Check sheet for the modelled part. Datum: model origin and axes. Units: mm. Face numbers are marked on the shaded views. A direction names the side the tool comes from. Give positions to 0.01 mm unless a question says otherwise; leave off trailing zeros. Order: outer loops, then holes, each group sorted by start corner. A loop starts at its lowest first (then second) coordinate and runs counter-clockwise, first axis right, second up. Notation, with made-up numbers: (36.5, -10) -> (40.5, -10) arc R19 cw to (40.5, -2) -> close; hole circle Ø3 at (6, -4.5). An arc over 180 degrees is marked (long way). Answer in a Markdown table with one row per item. Add a question column.
(1) Cross-section at D-D (x = 54). Record the cut outline in (y, z), then the cut area to 3 significant figures.
(2) Cross-section at B-B (x = 40). State how many separate pieces and enclosed holes the cut face has, then the cut area to 3 significant figures.
(3) Cross-section at C-C (y = 8). Record the cut outline in (x, z).
(4) Set-up check for the marked faces 1, 2, 3 and 4: record each of +Z, -Z, +X, -X, +Y, -Y from which the full face is reachable in a straight line by a thin tool's end or side.
(5) Thickness scan on L1, parallel to Z at x = 54, y = 13.25; L2, parallel to Z at x = 74, y = 1; L3, parallel to X at y = 5, z = 5. Record the ranges inside material, lowest first. Write a range as [from, to].
(6) Cross-section at A-A (z = 5). Record the cut outline in (x, y), then the cut area to 3 significant figures.
(7) Go/stop test with flat-tipped pins: pin 1 (5.5 mm diameter, centred on x = 30, z = -21.5, fed in from +Y); pin 2 (2 mm diameter, centred on x = 28, y = -36, fed in from -Z); pin 3 (3 mm diameter, centred on x = 74.5, z = -77, fed in from -Y); pin 4 (1.5 mm diameter, centred on x = 23.5, z = -4.5, fed in from -Y). Record where each tip stops, or that it passes through.
(8) Release check for a two-part mould opening along X. For the marked faces 5, 6 and 7 record: released by +X, released by -X, zero draft, split by the parting line, or undercut.
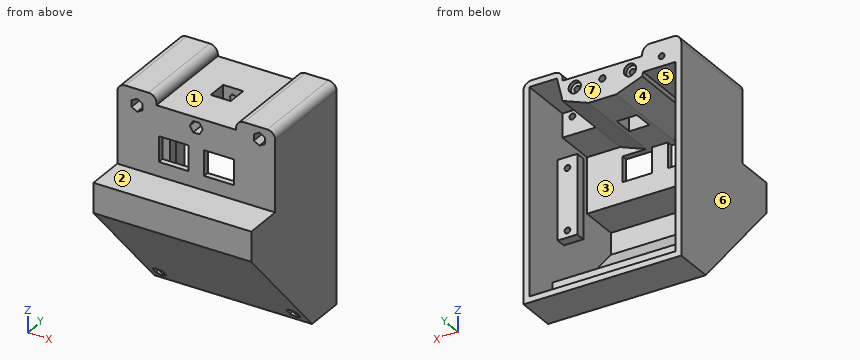
```python
from build123d import *

# Parameters (mm, degrees)
BOSS_EXTRUDE1_DEPTH = 80
SHELL1_T            = -3
SKETCH3_W           = 46
SKETCH3_H           = 47
BOSS_EXTRUDE2_DEPTH = 17
SKETCH4_W           = 10.2
SKETCH4_H           = 10.2
CUT_EXTRUDE1_DEPTH  = 20
SKETCH6_W           = 15
SKETCH6_H           = 12.8
CUT_EXTRUDE2_DEPTH  = 3
SKETCH7_W           = 40.4
SKETCH7_H           = 50
CUT_EXTRUDE3_DEPTH  = 5
FILLET1_R           = 4
CUT_EXTRUDE7_DEPTH  = 47
SKETCH13_R          = 1.5
CUT_EXTRUDE8_DEPTH  = 25
SKETCH14_R          = 3.1
CUT_EXTRUDE9_DEPTH  = 2
SKETCH17_W          = 45
SKETCH17_H          = 5
BOSS_EXTRUDE5_DEPTH = 74
CUT_EXTRUDE10_REACH = 48.51
SKETCH18_W          = 54
SKETCH18_H          = 45
CUT_EXTRUDE11_REACH = 48.51
SKETCH19_R          = 1.45
BOSS_EXTRUDE6_DEPTH = 47
SKETCH22_R          = 1.45
CUT_EXTRUDE12_DEPTH = 70.509632224
BOSS_EXTRUDE7_DEPTH = 74
SKETCH27_R          = 1.65
CUT_EXTRUDE14_DEPTH = 10
CUT_EXTRUDE15_START = -3
CUT_EXTRUDE15_DEPTH = 32
CUT_EXTRUDE16_DEPTH = 30
BOSS_EXTRUDE8_DEPTH = 20
SKETCH31_R          = 1.5
CUT_EXTRUDE17_DEPTH = 43.509632224
CUT_EXTRUDE18_DEPTH = 15
CUT_EXTRUDE19_REACH = 48.51
SKETCH33_W          = 10
SKETCH33_H          = 5
SKETCH34_R          = 1.6
CUT_EXTRUDE20_DEPTH = 70.509632224
CUT_EXTRUDE22_DEPTH = 14


with BuildPart() as part:
    # Sketch2 → Boss-Extrude1 (new body)
    with BuildSketch(Plane(origin=(0, 0, 0), x_dir=(0, 0, -1), z_dir=(1, 0, 0))):
        Polygon((-27.320490368, 20.998248687), (-27.320490368, -29.001751313), (12.679509632, -29.001751313), (12.679509632, -48.511383538), (27.679509632, -48.511383538), (82.679509632, 0.998248687), (82.679509632, 20.998248687), align=None)
    extrude(amount=BOSS_EXTRUDE1_DEPTH)

    # Shell1
    shell1_openings = [part.faces().sort_by_distance(p)[0] for p in [
        (40, 20.998248687, -27.679509632),
    ]]
    offset(amount=SHELL1_T, openings=shell1_openings, kind=Kind.INTERSECTION)

    # Sketch3 → Boss-Extrude2 (add)
    with BuildSketch(Plane(origin=(0, 0, 24.320490368), x_dir=(-1, 0, 0), z_dir=(0, 0, -1))):
        with Locations((-40, -2.501751313)):
            Rectangle(SKETCH3_W, SKETCH3_H)
    extrude(amount=BOSS_EXTRUDE2_DEPTH)

    # Sketch4 → Cut-Extrude1 (cut)
    with BuildSketch(Plane.XY.offset(27.320490368)):
        with Locations((40, -4.001751313)):
            Rectangle(SKETCH4_W, SKETCH4_H)
    extrude(amount=-CUT_EXTRUDE1_DEPTH, mode=Mode.SUBTRACT)

    # Sketch6 → Cut-Extrude2 (cut)
    with BuildSketch(Plane.XZ.offset(29.001751313)):
        with Locations((51.5, 0.920490368)):
            Rectangle(SKETCH6_W, SKETCH6_H)
        with Locations((28.5, 0.920490368)):
            Rectangle(SKETCH6_W, SKETCH6_H)
    extrude(amount=-CUT_EXTRUDE2_DEPTH, mode=Mode.SUBTRACT)

    # Sketch7 → Cut-Extrude3 (cut)
    with BuildSketch(Plane.XY.offset(27.320490368)):
        with Locations((40, -4.001751313)):
            Rectangle(SKETCH7_W, SKETCH7_H)
    extrude(amount=-CUT_EXTRUDE3_DEPTH, mode=Mode.SUBTRACT)

    # Fillet1
    fillet1_edges = [part.edges().sort_by_distance(p)[0] for p in [
        (19.8, -4.001751313, 27.320490368),
        (60.2, -4.001751313, 27.320490368),
        (80, -4.001751313, 27.320490368),
        (0, -4.001751313, 27.320490368),
    ]]
    fillet(fillet1_edges, radius=FILLET1_R)

    # Sketch12 → Cut-Extrude7 (cut)
    with BuildSketch(Plane(origin=(0, 20.998248687, 0), x_dir=(1, 0, 0), z_dir=(0, 1, 0))):
        Polygon((33, -7.320490368), (19.8, -12.320490368), (17, -24.320490368), (17, -7.320490368), align=None)
        Polygon((47, -7.320490368), (63, -7.320490368), (63, -24.320490368), (60.2, -12.320490368), align=None)
    extrude(amount=-CUT_EXTRUDE7_DEPTH, mode=Mode.SUBTRACT)

    # Sketch13 → Cut-Extrude8 (cut)
    with BuildSketch(Plane(origin=(0, 20.998248687, 0), x_dir=(1, 0, 0), z_dir=(0, 1, 0))):
        with Locations((26, -17.320490368)):
            Circle(SKETCH13_R)
        with Locations((54, -17.320490368)):
            Circle(SKETCH13_R)
    extrude(amount=-CUT_EXTRUDE8_DEPTH, mode=Mode.SUBTRACT)

    # Sketch14 → Cut-Extrude9 (cut)
    with BuildSketch(Plane(origin=(0, 20.998248687, 0), x_dir=(1, 0, 0), z_dir=(0, 1, 0))):
        with Locations((26, -17.320490368)):
            Circle(SKETCH14_R)
        with Locations((54, -17.320490368)):
            Circle(SKETCH14_R)
    extrude(amount=-CUT_EXTRUDE9_DEPTH, mode=Mode.SUBTRACT)

    # Sketch17 → Boss-Extrude5 (add)
    with BuildSketch(Plane.ZY.offset(-77)):
        with Locations((-23.179509632, -4.501751313)):
            Rectangle(SKETCH17_W, SKETCH17_H)
    extrude(amount=BOSS_EXTRUDE5_DEPTH)

    # Sketch18 → Cut-Extrude10 (cut, up to next)
    with BuildSketch(Plane(origin=(0, -2.001751313, 0), x_dir=(1, 0, 0), z_dir=(0, 1, 0)), mode=Mode.PRIVATE) as cut_extrude10_sk1:
        with Locations((40, 23.179509632)):
            Rectangle(SKETCH18_W, SKETCH18_H)
    cut_extrude10_tool1 = extrude(cut_extrude10_sk1.sketch, amount=-CUT_EXTRUDE10_REACH, mode=Mode.PRIVATE) & part.part
    add(cut_extrude10_tool1.solids().sort_by_distance((40, -2.001751, -23.17951))[0], mode=Mode.SUBTRACT)

    # Sketch19 → Cut-Extrude11 (cut, up to next)
    with BuildSketch(Plane(origin=(0, -2.001751313, 0), x_dir=(1, 0, 0), z_dir=(0, 1, 0)), mode=Mode.PRIVATE) as cut_extrude11_sk1:
        with Locations((72, 37.179509632)):
            Circle(SKETCH19_R)
    cut_extrude11_tool1 = extrude(cut_extrude11_sk1.sketch, amount=-CUT_EXTRUDE11_REACH, mode=Mode.PRIVATE) & part.part
    add(cut_extrude11_tool1.solids().sort_by_distance((72, -2.001751, -37.17951))[0], mode=Mode.SUBTRACT)
    # Sketch19 → Cut-Extrude11 (cut, up to next)
    with BuildSketch(Plane(origin=(0, -2.001751313, 0), x_dir=(1, 0, 0), z_dir=(0, 1, 0)), mode=Mode.PRIVATE) as cut_extrude11_sk2:
        with Locations((72, 6.179509632)):
            Circle(SKETCH19_R)
    cut_extrude11_tool2 = extrude(cut_extrude11_sk2.sketch, amount=-CUT_EXTRUDE11_REACH, mode=Mode.PRIVATE) & part.part
    add(cut_extrude11_tool2.solids().sort_by_distance((72, -2.001751, -6.17951))[0], mode=Mode.SUBTRACT)
    # Sketch19 → Cut-Extrude11 (cut, up to next)
    with BuildSketch(Plane(origin=(0, -2.001751313, 0), x_dir=(1, 0, 0), z_dir=(0, 1, 0)), mode=Mode.PRIVATE) as cut_extrude11_sk3:
        with Locations((8, 33.179509632)):
            Circle(SKETCH19_R)
    cut_extrude11_tool3 = extrude(cut_extrude11_sk3.sketch, amount=-CUT_EXTRUDE11_REACH, mode=Mode.PRIVATE) & part.part
    add(cut_extrude11_tool3.solids().sort_by_distance((8, -2.001751, -33.17951))[0], mode=Mode.SUBTRACT)
    # Sketch19 → Cut-Extrude11 (cut, up to next)
    with BuildSketch(Plane(origin=(0, -2.001751313, 0), x_dir=(1, 0, 0), z_dir=(0, 1, 0)), mode=Mode.PRIVATE) as cut_extrude11_sk4:
        with Locations((8, 6.179509632)):
            Circle(SKETCH19_R)
    cut_extrude11_tool4 = extrude(cut_extrude11_sk4.sketch, amount=-CUT_EXTRUDE11_REACH, mode=Mode.PRIVATE) & part.part
    add(cut_extrude11_tool4.solids().sort_by_distance((8, -2.001751, -6.17951))[0], mode=Mode.SUBTRACT)

    # Sketch21 → Boss-Extrude6 (add)
    with BuildSketch(Plane(origin=(0, -26.001751313, 0), x_dir=(1, 0, 0), z_dir=(0, 1, 0))):
        Polygon((3, -24.320490368), (3, -14.320490368), (19.333333333, -14.320490368), (17, -24.320490368), align=None)
    extrude(amount=BOSS_EXTRUDE6_DEPTH)

    # Sketch22 → Cut-Extrude12 (cut, through all)
    with BuildSketch(Plane(origin=(0, 20.998248687, 0), x_dir=(1, 0, 0), z_dir=(0, 1, 0))):
        with Locations((10, -19.320490368)):
            Circle(SKETCH22_R)
    extrude(amount=-CUT_EXTRUDE12_DEPTH, mode=Mode.SUBTRACT)

    # Sketch26 → Boss-Extrude7 (add)
    with BuildSketch(Plane(origin=(3, 0, 0), x_dir=(0, 0, -1), z_dir=(1, 0, 0))):
        Polygon((79.679509632, 2.334161996), (63.679509632, 2.334161996), (63.679509632, -12.068640106), align=None)
    extrude(amount=BOSS_EXTRUDE7_DEPTH)

    # Sketch27 → Cut-Extrude14 (cut)
    with BuildSketch(Plane(origin=(0, 2.334161996, 0), x_dir=(1, 0, 0), z_dir=(0, 1, 0))):
        with Locations((6, 76.679509632)):
            Circle(SKETCH27_R)
        with Locations((74, 76.679509632)):
            Circle(SKETCH27_R)
    extrude(amount=-CUT_EXTRUDE14_DEPTH, mode=Mode.SUBTRACT)

    # Sketch28 → Cut-Extrude15 (cut)
    with BuildSketch(Plane(origin=(0, 2.334161996, 0), x_dir=(1, 0, 0), z_dir=(0, 1, 0)).offset(CUT_EXTRUDE15_START)):
        Polygon((74, 79.929509632), (71.185417438, 78.304509632), (71.185417438, 75.054509632), (74, 73.429509632), (76.814582562, 75.054509632), (76.814582562, 78.304509632), align=None)
        Polygon((6, 73.429509632), (8.814582562, 75.054509632), (8.814582562, 78.304509632), (6, 79.929509632), (3.185417438, 78.304509632), (3.185417438, 75.054509632), align=None)
    extrude(amount=-CUT_EXTRUDE15_DEPTH, mode=Mode.SUBTRACT)

    # Sketch29 → Cut-Extrude16 (cut)
    with BuildSketch(Plane.XZ.offset(29.001751313)):
        Polygon((7.185417438, 17.695490368), (10, 16.070490368), (12.814582562, 17.695490368), (12.814582562, 20.945490368), (10, 22.570490368), (7.185417438, 20.945490368), align=None)
    extrude(amount=-CUT_EXTRUDE16_DEPTH, mode=Mode.SUBTRACT)

    # Sketch30 → Boss-Extrude8 (add)
    with BuildSketch(Plane(origin=(0, -26.001751313, 0), x_dir=(1, 0, 0), z_dir=(0, 1, 0))):
        Polygon((77, -24.320490368), (63, -24.320490368), (60.2, -12.320490368), (77, -12.320490368), align=None)
    extrude(amount=BOSS_EXTRUDE8_DEPTH)

    # Sketch31 → Cut-Extrude17 (cut, through all)
    with BuildSketch(Plane(origin=(0, -6.001751313, 0), x_dir=(1, 0, 0), z_dir=(0, 1, 0))):
        with Locations((72, -21.320490368)):
            Circle(SKETCH31_R)
    extrude(amount=-CUT_EXTRUDE17_DEPTH, mode=Mode.SUBTRACT)

    # Sketch32 → Cut-Extrude18 (cut)
    with BuildSketch(Plane.XZ.offset(29.001751313)):
        Polygon((72, 24.570490368), (69.185417438, 22.945490368), (69.185417438, 19.695490368), (72, 18.070490368), (74.814582562, 19.695490368), (74.814582562, 22.945490368), align=None)
    extrude(amount=-CUT_EXTRUDE18_DEPTH, mode=Mode.SUBTRACT)

    # Sketch33 → Cut-Extrude19 (cut, up to next)
    with BuildSketch(Plane(origin=(0, -2.001751313, 0), x_dir=(1, 0, 0), z_dir=(0, 1, 0)), mode=Mode.PRIVATE) as cut_extrude19_sk1:
        with Locations((72, 43.179509632)):
            Rectangle(SKETCH33_W, SKETCH33_H)
    cut_extrude19_tool1 = extrude(cut_extrude19_sk1.sketch, amount=-CUT_EXTRUDE19_REACH, mode=Mode.PRIVATE) & part.part
    add(cut_extrude19_tool1.solids().sort_by_distance((72, -2.001751, -43.17951))[0], mode=Mode.SUBTRACT)

    # Sketch34 → Cut-Extrude20 (cut, through all)
    with BuildSketch(Plane(origin=(0, 20.998248687, 0), x_dir=(1, 0, 0), z_dir=(0, 1, 0))):
        with Locations((40, -17.320490368)):
            Circle(SKETCH34_R)
    extrude(amount=-CUT_EXTRUDE20_DEPTH, mode=Mode.SUBTRACT)

    # Sketch36 → Cut-Extrude22 (cut)
    with BuildSketch(Plane.XZ.offset(29.001751313)):
        Polygon((38.375, 20.13507293), (36.75, 17.320490368), (38.375, 14.505907805), (41.625, 14.505907805), (43.25, 17.320490368), (41.625, 20.13507293), align=None)
    extrude(amount=-CUT_EXTRUDE22_DEPTH, mode=Mode.SUBTRACT)


solid = part.part
```
Answer below:
| question | item | result |
|---|---|---|
| 1 | outline | (-48.51, -27.68) -> (1, -82.68) -> (21, -82.68) -> (21, -79.68) -> (2.33, -79.68) -> (2.33, -63.68) -> (-12.07, -63.68) -> (-45.51, -26.53) -> (-45.51, -15.68) -> (-26, -15.68) -> (-26, -5.48) -> (-29, -5.48) -> (-29, -12.68) -> (-48.51, -12.68) -> close; (-29, 7.32) -> (-26, 7.32) -> (-26, 9.97) -> (21, 9.97) -> (21, 14.22) -> (19, 14.22) -> (19, 15.82) -> (-4, 15.82) -> (-4, 18.82) -> (19, 18.82) -> (19, 20.42) -> (21, 20.42) -> (21, 22.32) -> (-29, 22.32) -> close |
| 1 | area | 1,060 mm² |
| 2 | separate pieces | 4 |
| 2 | enclosed holes | 0 |
| 2 | area | 989 mm² |
| 3 | outline | (0, -82.68) -> (80, -82.68) -> (80, 23.32) arc R4 ccw to (76, 27.32) -> (64.2, 27.32) arc R4 ccw to (60.2, 23.32) -> (60.2, 22.32) -> (19.8, 22.32) -> (19.8, 23.32) arc R4 ccw to (15.8, 27.32) -> (4, 27.32) arc R4 ccw to (0, 23.32) -> close; hole (3, -79.68) -> (77, -79.68) -> (77, 24.32) -> (63, 24.32) -> (60.2, 12.32) -> (47, 7.32) -> (33, 7.32) -> (19.8, 12.32) -> (19.33, 14.32) -> (3, 14.32) -> close; hole circle Ø2.9 at (10, 19.32); hole circle Ø3 at (26, 17.32); hole circle Ø3.2 at (40, 17.32); hole circle Ø3 at (54, 17.32) |
| 4 | face 1 | +Z, +Y, -Y |
| 4 | face 2 | +Z, +X, -X, -Y |
| 4 | face 3 | none |
| 4 | face 4 | +Y |
| 5 | L1 | z = [-82.68, -79.68], [9.97, 15.82], [18.82, 22.32] |
| 5 | L2 | z = [-82.68, -78.33], [-75.03, -63.68], [24.32, 27.32] |
| 5 | L3 | x = [0, 3], [77, 80] |
| 6 | outline | (0, -29) -> (21, -29) -> (21, -26) -> (3, -26) -> (3, 21) -> (0, 21) -> close; (36, -29) -> (44, -29) -> (44, -26) -> (36, -26) -> close; (59, -29) -> (80, -29) -> (80, 21) -> (77, 21) -> (77, -26) -> (59, -26) -> close |
| 6 | area | 432 mm² |
| 7 | pin 1 | stops at y = -45.51 |
| 7 | pin 2 | stops at z = -42.69 |
| 7 | pin 3 | stops at y = -0.67 |
| 7 | pin 4 | passes through |
| 8 | face 5 | undercut |
| 8 | face 6 | released by -X |
| 8 | face 7 | zero draft |
